Input: dimensioned drawing with shaded views. Units: mm. Origin: part minimum x, y, z. A direction names the side the tool comes from. Coordinates: 2 decimals unless noted, no trailing zeros. Loops run counter-clockwise (first coordinate to the right, second up) from the corner with the lowest first, then second, coordinate; pieces in that order, holes last. Notation, with made-up numbers: (-23, 85) - (7, 85) arc R21 cw to (7, 119) - close; hole circle Ø9 at (-15.75, 26). An arc over 180 degrees is marked (long way). Write item = value, one per line. Start each with the question number.
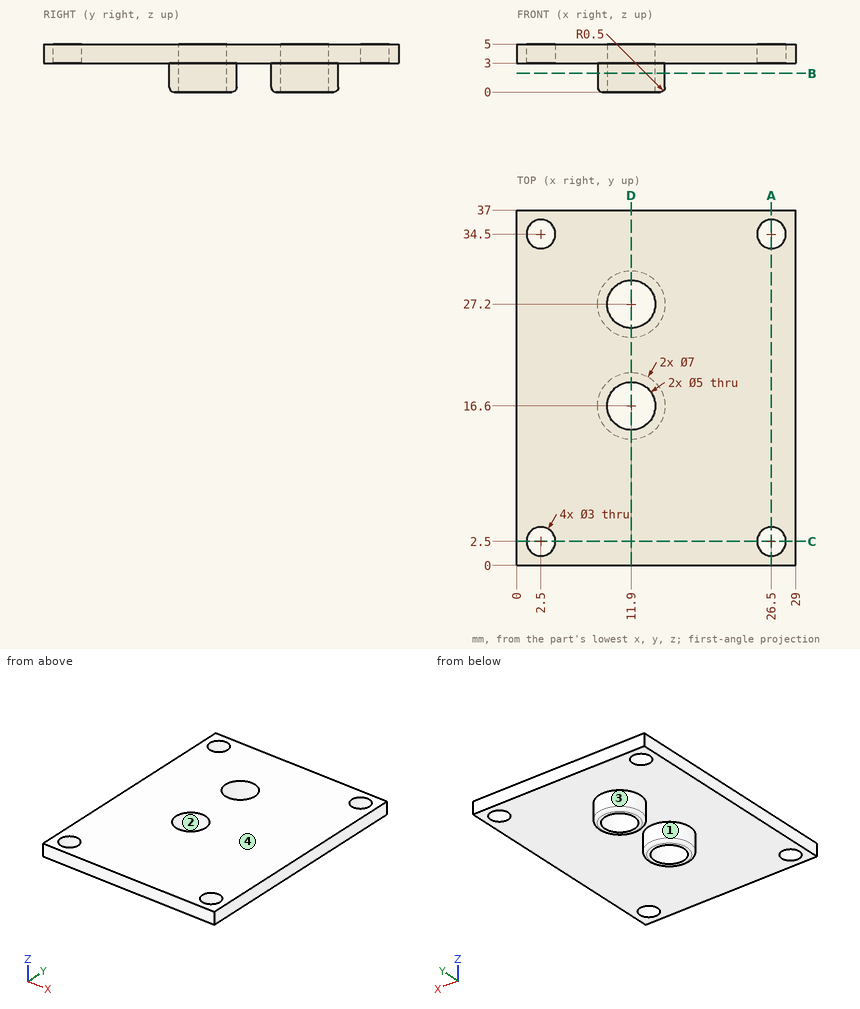
Item 1: Ray query, line 1 (Y direction, x = 2.5, z = 3.75); line 2 (Y direction, x = 11.9, z = 2.15); line 3 (Z direction, x = 14.25, y = 11.5). Return the intervals inside material, ascending.
Item 2: Cut plane B-B on z = 1.95. Return loops of the section in (x, y).
Item 3: Cut plane A-A on x = 26.5. Return loops of the section in (y, z), plus the area to 3 significant figures.
Item 4: Pin query (flat end, axial travel): pin 1 (5 mm diameter, centred on x = 12.5, y = 26.5, fed in from -Z); pin 2 (1 mm diameter, centred on x = 8, y = 11, fed in from -Z). Return the tip coordinate at first contact, or that it passes through.
Item 5: Cut plane C-C on y = 2.5. Return loops of the section in (x, z).
Item 6: Access query for the marked faces 1 and 2. Directions: +Z, -Z, +X, -X, +Y, -Y. A direction counts if a zero-diameter tool reaches every point of the face in a straight line with its end or side. Return the directions, or none.
Item 7: Cut plane D-D on x = 11.9. Return loops of the section in (y, z), plus the area to 3 significant figures.
Item 8: Pull-direction query (Y, two-part tool) for the marked faces 3 and 4; classes: pulls with the +Y half, pulls with the -Y half, needs draft (parallel to the pull), parting line crosses it, or undercut.
Recorded:
q1.line_1 = 0 to 1, 4 to 33, 36 to 37
q1.line_2 = 13.1 to 14.1, 19.1 to 20.1, 23.7 to 24.7, 29.7 to 30.7
q1.line_3 = 3 to 5
q2.outline = circle Ø7 at (11.9, 16.6); circle Ø7 at (11.9, 27.2); hole circle Ø5 at (11.9, 16.6); hole circle Ø5 at (11.9, 27.2)
q3.outline = (0, 3) - (1, 3) - (1, 5) - (0, 5) - close; (4, 3) - (33, 3) - (33, 5) - (4, 5) - close; (36, 3) - (37, 3) - (37, 5) - (36, 5) - close
q3.area = 62.0 mm²
q4.pin_1 = 0
q4.pin_2 = 3
q5.outline = (0, 3) - (1, 3) - (1, 5) - (0, 5) - close; (4, 3) - (25, 3) - (25, 5) - (4, 5) - close; (28, 3) - (29, 3) - (29, 5) - (28, 5) - close
q6.face_1 = -Z
q6.face_2 = +Z, -Z
q7.outline = (0, 3) - (13.1, 3) - (13.1, 0.5) arc R0.5 ccw to (13.6, 0) - (14.1, 0) - (14.1, 5) - (0, 5) - close; (19.1, 0) - (19.6, 0) arc R0.5 ccw to (20.1, 0.5) - (20.1, 3) - (23.7, 3) - (23.7, 0.5) arc R0.5 ccw to (24.2, 0) - (24.7, 0) - (24.7, 5) - (19.1, 5) - close; (29.7, 0) - (30.2, 0) arc R0.5 ccw to (30.7, 0.5) - (30.7, 3) - (37, 3) - (37, 5) - (29.7, 5) - close
q7.area = 65.8 mm²
q8.face_3 = undercut
q8.face_4 = needs draft
